Input: part model. Units: mm. Frame: model coordinates. Face numbers are marked on the shaded views. A direction names the side the tool comes from. Give positions to 0.01 mm unless a question says otherwise; leave off trailing zeros. Loops run counter-clockwise (first coordinate to the right, second up) from the corner with the lowest first, then second, coordinate; pieces in that order, holes last. Notation, with made-up numbers: (75, 58) - (132, 58) arc R30 ccw to (132, 88) - close; hole circle Ø7 at (14, -29.5). An arc over 180 degrees is marked (long way). Answer as a JSON object with one key per item and string values. Group by question number.
(1) Section query C-C (y = -20). Return loops of the section in (x, z).
(2) Section query A-A (x = 0). Return loops of the section in (y, z), plus the area to 3 significant figures.
(3) Pin query (flat end, axial travel): P1, Ø19, axis at y = -16, z = 29, coming from the -X side; P2, Ø3, axis at x = 5.5, y = -1, coming from the +Z side; P3, Ø5, axis at x = 0, y = 20, coming from the +Z side. Return the tip coordinate at first contact, or that it passes through.
(4) Section query B-B (z = 20). Return loops of the section in (x, y), plus the area to 3 significant figures.
(5) Material intervals for L1, parallel to Y at x = 0, z = 1; L2, parallel to Z at x = 19, y = 20; L3, parallel to X at y = 3, z = 26, sorted ascending.
(6) Section query D-D (y = 9). Return loops of the section in (x, z).
(7) Access query for the marked faces 1 and 2. Directions: +Z, -Z, +X, -X, +Y, -Y. A direction counts if a zero-diameter tool reaches every point of the face in a straight line with its end or side. Return the directions, or none.
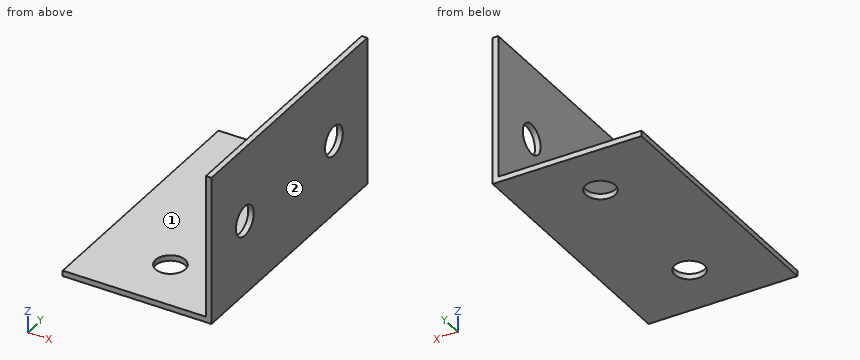
```python
from build123d import *

# Parameters (mm, degrees)
SZKIC1_W                    = 40
SZKIC1_H                    = 70
DODANIE_WYCI_GNI_CIE1_DEPTH = 40
SZKIC2_W                    = 38.5
SZKIC2_H                    = 38.5
WYTNIJ_WYCI_GNI_CIE1_DEPTH  = 80
SZKIC3_R                    = 4
WYTNIJ_WYCI_GNI_CIE2_DEPTH  = 80
SZKIC11_R                   = 4
WYTNIJ_WYCI_GNI_CIE3_DEPTH  = 40


with BuildPart() as part:
    # Szkic1 → Dodanie-wyciągnięcie1 (new body)
    with BuildSketch(Plane.XY):
        Rectangle(SZKIC1_W, SZKIC1_H)
    extrude(amount=DODANIE_WYCI_GNI_CIE1_DEPTH)

    # Szkic2 → Wytnij-wyciągnięcie1 (cut)
    with BuildSketch(Plane(origin=(0, 35, 0), x_dir=(1, 0, 0), z_dir=(0, 1, 0))):
        with Locations((-0.75, -20.75)):
            Rectangle(SZKIC2_W, SZKIC2_H)
    extrude(amount=-WYTNIJ_WYCI_GNI_CIE1_DEPTH, mode=Mode.SUBTRACT)

    # Szkic3 → Wytnij-wyciągnięcie2 (cut)
    with BuildSketch(Plane.ZY.offset(-18.5)):
        with Locations(Location((20, 20, 0), (0, 0, 270))):
            Circle(SZKIC3_R)
        with Locations((20, -20)):
            Circle(SZKIC3_R)
    extrude(amount=-WYTNIJ_WYCI_GNI_CIE2_DEPTH, mode=Mode.SUBTRACT)

    # Szkic11 → Wytnij-wyciągnięcie3 (cut)
    with BuildSketch(Plane.XY.offset(1.5)):
        with Locations((0, 20)):
            Circle(SZKIC11_R)
        with Locations((0, -20)):
            Circle(SZKIC11_R)
    extrude(amount=-WYTNIJ_WYCI_GNI_CIE3_DEPTH, mode=Mode.SUBTRACT)


solid = part.part
```
Recorded:
{
 "1": {"outline": "(-20, 0) - (-4, 0) - (-4, 1.5) - (-20, 1.5) - close; (4, 0) - (20, 0) - (20, 16) - (18.5, 16) - (18.5, 1.5) - (4, 1.5) - close; (18.5, 24) - (20, 24) - (20, 40) - (18.5, 40) - close"},
 "2": {"outline": "(-35, 0) - (-24, 0) - (-24, 1.5) - (-35, 1.5) - close; (-16, 0) - (16, 0) - (16, 1.5) - (-16, 1.5) - close; (24, 0) - (35, 0) - (35, 1.5) - (24, 1.5) - close", "area": "81.0 mm^2"},
 "3": {"P1": "stops at x = 18.5", "P2": "stops at z = 1.5", "P3": "passes through"},
 "4": {"outline": "(18.5, -35) - (20, -35) - (20, -24) - (18.5, -24) - close; (18.5, -16) - (20, -16) - (20, 16) - (18.5, 16) - close; (18.5, 24) - (20, 24) - (20, 35) - (18.5, 35) - close", "area": "81.0 mm^2"},
 "5": {"L1": "y = -35 to -24, -16 to 16, 24 to 35", "L2": "z = 0 to 16, 24 to 40", "L3": "x = 18.5 to 20"},
 "6": {"outline": "(-20, 0) - (20, 0) - (20, 40) - (18.5, 40) - (18.5, 1.5) - (-20, 1.5) - close"},
 "7": {"face 1": "+Z, -X, +Y, -Y", "face 2": "+Z, -Z, +X, +Y, -Y"}
}
